The listing builds one solid part. Answer for the finished solid, in the listing's coordinates (mm). A direction names the side the tool comes from. Round coordinates to 2 decimals unless told otherwise and drop trailing zeros. Order: outer loops, then holes, each group sorted by start corner. A loop starts at its lowest first (then second) coordinate and runs counter-clockwise, first axis right, second up. Notation, with made-up numbers: (-16.75, 25.25) - (29.25, 25.25) arc R9 cw to (29.25, 32.25) - close; hole circle Ø8 at (89, 80). An arc over 180 degrees is marked (long way). Use CSV: the item, a comma, the result in double quotes. Start each with the question number.
Item 1: Find section D-D, the plane z = 2.7. Count the separate pieces of the cut face and the enclosed holes in it, plus the area to 3 significant figures.
Item 2: Find section C-C, the plane x = 25. Give the vertices of the cut face in (y, z), plus the area to 3 significant figures.
Item 3: Determine the mould class of faces 1 (the flat face through (48, -10, 2)), 2 (the flat face through (28, -42.5, 2)), 3 (the flat face through (-35, 41, 2)) for opening direction Y: +Y half, -Y half, draft (parallel to the pull), parting line (faces both ways), or undercut.
Item 4: Find section A-A, the plane y = 15.1. Give the vertices of the cut face in (x, z), plus the area to 3 significant figures.
Item 5: For faces 4 (the flat face through (20, -41, 2)), 5 (the flat face through (-46.8, 0, 2)), 6 (the flat face through (-48, 25, 2)), determine the directions among +Z, -Z, +X, -X, +Y, -Y from which every point of the face is accessible in a straight line to the end or side of a thin tool.
Item 6: Flat-ended cylindrical pins translate along their axes: P1, Ø1.6, axis at y = 34.5, z = 2, coming from the -X side; P2, Ø1.6, axis at y = 41.5, z = 1, coming from the -X side; P3, Ø1, axis at x = 48, z = 2, coming from the -Y side; P4, Ø2.5, axis at x = 25, y = 15.1, coming from the -Z side. Find the tip coordinate at first contact, or state that the pin passes through.
Item 7: Straight lines are drawn through the part: line 1 along Y through (x, z) = (-25, 2.4); line 2 along X through (y, z) = (-12.5, 1.8); line 3 along X through (y, z) = (22.5, 0.9). For each, find the intervals that lie inside material, in ascending order. Write a range as [from, to].
Item 8: Find section B-B, the plane x = -13. Give the vertices of the cut face in (y, z).
```python
from build123d import *

# Parameters (mm, degrees)
SKETCH1_R           = 8
SKETCH1_R_2         = 3
SKETCH1_R_3         = 1.49
BOSS_EXTRUDE1_DEPTH = 3.2


with BuildPart() as part:
    # Sketch1 → Boss-Extrude1 (new body)
    with BuildSketch(Plane.XY):
        Polygon((-50, 10), (-50, 25), (-46.8, 25), (-46.8, 39.3), (-35, 39.3), (-35, 42.5), (-20, 42.5), (-20, 39.3), (-7.5, 39.3), (-7.5, 42.5), (7.5, 42.5), (7.5, 39.3), (20, 39.3), (20, 42.5), (35, 42.5), (35, 39.3), (46.8, 39.3), (46.8, 25), (50, 25), (50, 10), (46.8, 10), (46.8, -10), (50, -10), (50, -25), (46.8, -25), (46.8, -39.3), (35, -39.3), (35, -42.5), (20, -42.5), (20, -39.3), (7.5, -39.3), (7.5, -42.5), (-7.5, -42.5), (-7.5, -39.3), (-20, -39.3), (-20, -42.5), (-35, -42.5), (-35, -39.3), (-46.8, -39.3), (-46.8, -25), (-50, -25), (-50, -10), (-46.8, -10), (-46.8, 10), align=None)
        with Locations((-13, -8)):
            Circle(SKETCH1_R, mode=Mode.SUBTRACT)
        with Locations((-25, 20)):
            Circle(SKETCH1_R_2, mode=Mode.SUBTRACT)
        with Locations((-25, 15.1)):
            Circle(SKETCH1_R_3, mode=Mode.SUBTRACT)
        with Locations((13, -8)):
            Circle(SKETCH1_R, mode=Mode.SUBTRACT)
        with Locations((25, 15.1)):
            Circle(SKETCH1_R_3, mode=Mode.SUBTRACT)
        with Locations((25, 20)):
            Circle(SKETCH1_R_2, mode=Mode.SUBTRACT)
    extrude(amount=BOSS_EXTRUDE1_DEPTH)


solid = part.part
```
Worked out:
1,separate pieces,"1"
1,enclosed holes,"6"
1,area,"7,360 mm²"
2,outline,"(-42.5, 0) - (13.61, 0) - (13.61, 3.2) - (-42.5, 3.2) - close; (16.59, 0) - (17, 0) - (17, 3.2) - (16.59, 3.2) - close; (23, 0) - (42.5, 0) - (42.5, 3.2) - (23, 3.2) - close"
2,area,"243 mm²"
3,face 1,"undercut"
3,face 2,"-Y half"
3,face 3,"draft"
4,outline,"(-50, 0) - (-26.49, 0) - (-26.49, 3.2) - (-50, 3.2) - close; (-23.51, 0) - (23.51, 0) - (23.51, 3.2) - (-23.51, 3.2) - close; (26.49, 0) - (50, 0) - (50, 3.2) - (26.49, 3.2) - close"
4,area,"301 mm²"
5,face 4,"+Z, -Z, -Y"
5,face 5,"+Z, -Z, -X"
5,face 6,"+Z, -Z, -X, +Y"
6,P1,"stops at x = -46.8"
6,P2,"stops at x = -35"
6,P3,"stops at y = -25"
6,P4,"passes through"
7,line 1,"y = [-42.5, 13.61], [16.59, 17], [23, 42.5]"
7,line 2,"x = [-50, -19.61], [-6.39, 6.39], [19.61, 50]"
7,line 3,"x = [-50, -26.66], [-23.34, 23.34], [26.66, 50]"
8,outline,"(-39.3, 0) - (-16, 0) - (-16, 3.2) - (-39.3, 3.2) - close; (0, 0) - (39.3, 0) - (39.3, 3.2) - (0, 3.2) - close"
